Source: CAD feature listing. Evaluate the final solid. Frame: model axes, mm. Face numbers are marked on the shaded views. A direction names the side the tool comes from. Round coordinates to 2 decimals unless told otherwise and drop trailing zeros. Loops run counter-clockwise (first coordinate to the right, second up) from the corner with the lowest first, then second, coordinate; pieces in that order, holes last. Notation, with made-up numbers: M 8.5,-35.75 L 25.5,-35.75 A22 ccw 25.5,-29.75 Z; hole C -8,-33.75 d6. An arc over 180 degrees is marked long. Answer as a JSON object with one key per item and string values.
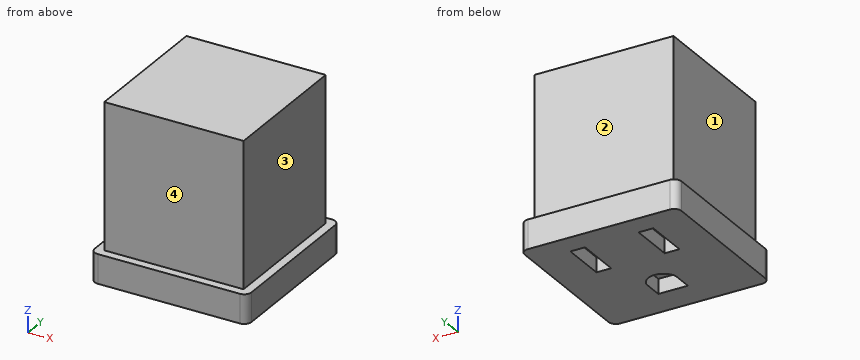
from build123d import *

# Parameters (mm, degrees)
SKETCH1_W           = 27
SKETCH1_H           = 27
BOSS_EXTRUDE1_DEPTH = 5
SKETCH2_W           = 24
SKETCH2_H           = 24
BOSS_EXTRUDE2_DEPTH = 25
FILLET1_R           = 1.27
SKETCH3_W           = 2.54
SKETCH3_H           = 7.62
CUT_EXTRUDE1_DEPTH  = 2.54


with BuildPart() as part:
    # Sketch1 → Boss-Extrude1 (new body)
    with BuildSketch(Plane.XY):
        with Locations((13.5, 13.5)):
            Rectangle(SKETCH1_W, SKETCH1_H)
    extrude(amount=BOSS_EXTRUDE1_DEPTH)

    # Sketch2 → Boss-Extrude2 (add)
    with BuildSketch(Plane.XY.offset(5)):
        with Locations((13.5, 13.5)):
            Rectangle(SKETCH2_W, SKETCH2_H)
    extrude(amount=BOSS_EXTRUDE2_DEPTH)

    # Fillet1
    fillet1_edges = [part.edges().sort_by_distance(p)[0] for p in [
        (0, 27, 2.5),
        (27, 27, 2.5),
        (27, 0, 2.5),
        (0, 0, 2.5),
    ]]
    fillet(fillet1_edges, radius=FILLET1_R)

    # Sketch3 → Cut-Extrude1 (cut)
    with BuildSketch(Plane(origin=(0, 0, 0), x_dir=(-1, 0, 0), z_dir=(0, 0, -1))):
        with Locations((-19.38, 19.38)):
            Rectangle(SKETCH3_W, SKETCH3_H)
        with Locations((-7.62, 19.38)):
            Rectangle(SKETCH3_W, SKETCH3_H)
        with BuildLine():
            Line((-16.164953657, 5.08), (-16.164953657, 8.636))
            ThreePointArc((-16.164953657, 8.636), (-13.624953657, 10.494493494), (-11.084953657, 8.636))
            Line((-11.084953657, 8.636), (-11.084953657, 5.08))
            Line((-11.084953657, 5.08), (-16.164953657, 5.08))
        make_face()
    extrude(amount=-CUT_EXTRUDE1_DEPTH, mode=Mode.SUBTRACT)


solid = part.part
Item 1: Section B-B on y = 13.25. Return the cut outline in (x, z), then the cut area to 3 significant figures.
Answer sheet:
{"outline": "M 0,0 L 27,0 L 27,5 L 25.5,5 L 25.5,30 L 1.5,30 L 1.5,5 L 0,5 Z", "area": "735 mm²"}
Item 2: Line query: probe 1 along X at (y, z) = (8, 9); probe 2 along Z at (x, y) = (14.75, 10). Output: solid intervals per line, ascending. Write a range as from..to.
Answer sheet:
{"probe 1": "x = 1.5..25.5", "probe 2": "z = 2.54..30"}
Item 3: Section C-C on z = 16. Return the cut outline in (x, y), then the cut area to 3 significant figures.
Answer sheet:
{"outline": "M 1.5,1.5 L 25.5,1.5 L 25.5,25.5 L 1.5,25.5 Z", "area": "576 mm²"}
Item 4: Section A-A on x = 19. Return the cut outline in (y, z), then the cut area to 3 significant figures.
Answer sheet:
{"outline": "M 0,0 L 15.57,0 L 15.57,2.54 L 23.19,2.54 L 23.19,0 L 27,0 L 27,5 L 25.5,5 L 25.5,30 L 1.5,30 L 1.5,5 L 0,5 Z", "area": "716 mm²"}
Item 5: Access query for the marked faces 1, 2, 3 and 4. Directions: +Z, -Z, +X, -X, +Y, -Y. A direction counts if a zero-diameter tool reaches every point of the face in a straight line with its end or side. Return the directions, or none.
Answer sheet:
{"face 1": "+Z, -X, +Y, -Y", "face 2": "+Z, +X, -X, +Y", "face 3": "+Z, +X, +Y, -Y", "face 4": "+Z, +X, -X, -Y"}
Item 6: Contact query for flat-ended pins moving along their axis: pin 1 Ø5 at (x, z) = (4, 21) entering from -Y; pin 2 Ø6 at (y, z) = (7.5, 16) entering from +X; pin 3 Ø2 at (x, y) = (7.5, 21) entering from -Z. Output: stop coordinate, or through.
Answer sheet:
{"pin 1": "stops at y = 1.5", "pin 2": "stops at x = 25.5", "pin 3": "stops at z = 2.54"}
